Answer from the drawing. Dimensions are ordinates in mm from the lowest x, y and z of the part. Give positions to 0.01 mm unless a question says otherwise; leave off trailing zeros. Loops run counter-clockwise (first coordinate to the right, second up) from the corner with the lowest first, then second, coordinate; pieces in that order, holes last. Notation, with made-up numbers: (7.5, 14) -> (63.5, 14) arc R15 ccw to (63.5, 31) -> close; hole circle Ø11 at (57.5, 22). An arc over 180 degrees is marked (long way). Return JSON: item names as keys, results as strings. Group by question number.
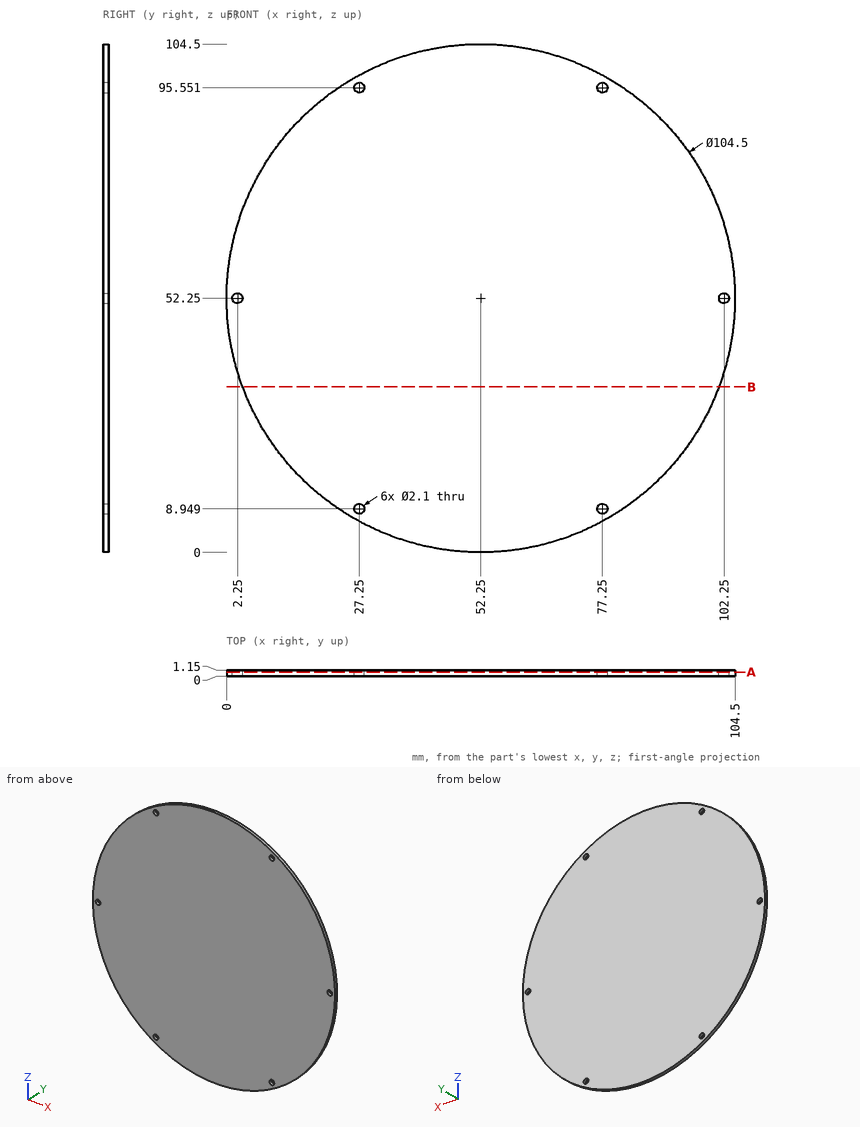
1. Section B-B on z = 34 is taken. Determine the outline of the cut face in (x, y).
2. Section A-A on y = 0.8 is taken. Determine the outline of the cut face in (x, z).
3. Straight lines are drawn through the part: line 1 (X direction, y = 0.55, z = 52.25); line 2 (Z direction, x = 27.25, y = 0.5); line 3 (X direction, y = 0.15, z = 6.5). For each, find the intervals that lie inside material, in ascending order. Write a range as from..to.
Completed:
{
 "1": {"outline": "(3.29, 0) -> (101.21, 0) -> (101.21, 1.15) -> (3.29, 1.15) -> close"},
 "2": {"outline": "circle Ø104.5 at (52.25, 52.25); hole circle Ø2.1 at (2.25, 52.25); hole circle Ø2.1 at (27.25, 8.95); hole circle Ø2.1 at (27.25, 95.55); hole circle Ø2.1 at (77.25, 8.95); hole circle Ø2.1 at (77.25, 95.55); hole circle Ø2.1 at (102.25, 52.25)"},
 "3": {"line 1": "x = 0..1.2, 3.3..101.2, 103.3..104.5", "line 2": "z = 6.37..7.9, 10..94.5, 96.6..98.13", "line 3": "x = 27.01..77.49"}
}
